Verification items for the finished model (mm, model axes). Face numbers are marked on the shaded views. A direction names the side the tool comes from. Give positions to 0.01 mm unless a question says otherwise; leave off trailing zeros. Order: outer loops, then holes, each group sorted by start corner. A loop starts at its lowest first (then second) coordinate and runs counter-clockwise, first axis right, second up.
(1) Sectioned sample at C-C on z = 38. Record the cut outline in (x, y).
(2) Sectioned sample at D-D on y = -10. Record the cut outline in (x, z).
(3) Scan lines: L1, parallel to Y at x = 0, z = 2.9; L2, parallel to Z at x = 3, y = 20.5; L3, parallel to Y at x = 2, z = 17. Record each from-to range of solid material in increasing order.
(4) Access from +Z, -Z, +X, -X, +Y, -Y to the whole of each face (thin tool, end or side, straight path). Record for the marked faces 1, 2, 3, 4 and 5.
(5) Sectioned sample at B-B on x = 0. Record the cut outline in (y, z), plus the area to 3 significant figures.
(6) Sectioned sample at A-A on y = 20. Record the cut outline in (x, z).
(7) Gauge pin test, flat ends, axial feed: pin 1 (1.5 mm diameter, centred on y = 13.5, z = 8, fed in from +X); pin 2 (1.5 mm diameter, centred on y = -21, z = 30, fed in from +X); pin 3 (8 mm diameter, centred on x = 7, y = -3, fed in from +Z). Record the tip position at first contact, or that the pin passes through.
```python
from build123d import *

# Parameters (mm, degrees)
F0_R     = 25
F0_R_2   = 1.7
F1_DEPTH = 5
F3_W     = 6
F3_H     = 3
F4_DEPTH = 50


# Not quite as in the source:
# - a feature names something its author has since deleted; it is built from what else it names


with BuildPart() as f1:
    # F0 (on Top) → F1 (new body)
    with BuildSketch(Plane.XY):
        Circle(F0_R)
        with Locations((-17.3205080757, -10)):
            Circle(F0_R_2, mode=Mode.SUBTRACT)
        with Locations((17.3205080757, -10)):
            Circle(F0_R_2, mode=Mode.SUBTRACT)
        with Locations((0, 20)):
            Circle(F0_R_2, mode=Mode.SUBTRACT)
    extrude(amount=F1_DEPTH)

    # F3 (on face) → F4 (join)
    with BuildSketch(Plane.XY.offset(5)):
        Polygon((-16.6554445662, 6.1519237886), (-13.6554445662, 11.3480762114), (-16.2535207776, 12.8480762114), (-19.2535207776, 7.6519237886), align=None)
        Polygon((16.2017059222, 12.9378221735), (13.6036297108, 11.4378221735), (16.6036297108, 6.2416697508), (19.2017059222, 7.7416697508), align=None)
        with Locations((0, -21.5)):
            Rectangle(F3_W, F3_H)
    extrude(amount=F4_DEPTH)


solid = f1.part
```
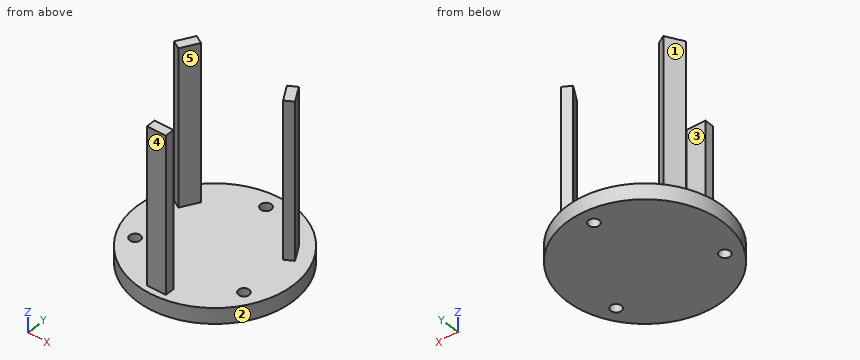
Ans:
1. outline: (-19.25, 7.65) - (-16.66, 6.15) - (-13.66, 11.35) - (-16.25, 12.85) - close; (-3, -23) - (3, -23) - (3, -20) - (-3, -20) - close; (13.6, 11.44) - (16.6, 6.24) - (19.2, 7.74) - (16.2, 12.94) - close
2. outline: (-22.91, 0) - (-19.02, 0) - (-19.02, 5) - (-22.91, 5) - close; (-15.62, 0) - (15.62, 0) - (15.62, 5) - (-15.62, 5) - close; (19.02, 0) - (22.91, 0) - (22.91, 5) - (19.02, 5) - close
3. L1: y = -25 to 18.3, 21.7 to 25
3. L2: z = 0 to 5
3. L3: y = -23 to -20
4. face 1: +Z, -X, +Y
4. face 2: +Z, -Z
4. face 3: +Z, +X, -X, +Y
4. face 4: +Z, +X, -X, -Y
4. face 5: +Z, -Y
5. outline: (-25, 0) - (18.3, 0) - (18.3, 5) - (-20, 5) - (-20, 55) - (-23, 55) - (-23, 5) - (-25, 5) - close; (21.7, 0) - (25, 0) - (25, 5) - (21.7, 5) - close
5. area: 383 mm2
6. outline: (-15, 0) - (-1.7, 0) - (-1.7, 5) - (-15, 5) - close; (1.7, 0) - (15, 0) - (15, 5) - (1.7, 5) - close
7. pin 1: stops at x = 16.31
7. pin 2: stops at x = 3
7. pin 3: stops at z = 5
